The model under review builds one solid part; all positions refer to its coordinate system, in mm. A direction names the side the tool comes from. Give positions to 0.01 mm unless a question says otherwise; leave off trailing zeros. Loops run counter-clockwise (first coordinate to the right, second up) from the corner with the lowest first, then second, coordinate; pieces in that order, holes last. Notation, with made-up numbers: M 10,-28.5 L 16,-28.5 A16 cw 16,-1.5 Z; hole C 77,66.25 d11. An arc over 180 degrees is marked long. One line per item, written item: value. Start each with the question number.
Q1. We need section B-B on x = -7. Write out the cut boundary in (y, z).
Q2. We need section A-A on x = 0. Write out the cut boundary in (y, z).
Q3. For faces 4 (the face through (-10.011, 0.74, 10.124)), 5 (the face through (4.052, 4.986, -2.324)), 6 (the face through (-4.032, 3, 0)), list the 3-axis set-ups (+Z, -Z, +X, -X, +Y, -Y) from which the entire face can be reached by the end or side of a thin tool; tool diameter is ignored.
Q4. We need section D-D on x = 15. Write out the cut boundary in (y, z), plus the area to 3 significant figures.
Q5. To check wall thickness, follow line 1 along Y through (x, z) = (-4, 0.5); line 2 along X through (y, z) = (0.7, 8.5); line 3 along Y through (x, z) = (19, 9.5). State the ranges of each line that lie inside material, in increasing order. Write a range as from..to.
Q6. For pin 1 (1 mm diameter, centred on x = 19.5, z = -9, fed in from -Y); pin 2 (0.6 mm diameter, centred on y = 5.5, z = -2.5, fed in from -X); pin 3 (1 mm diameter, centred on y = 4.5, z = 8.5, fed in from +X); pin 4 (1 mm diameter, centred on x = -6.5, y = 4.5, fed in from -Z), all flat-tipped, find the tip position at first contact; note any pin that passes through.
Q7. Mouldability with a two-part tool opening along X and no side actions: class faces 1 (the face through (0, 1, -11.5)), 2 (the face through (3.815, 4.986, 3.181)), 3 (the face through (5.098, 5, 0)) as released by +X, released by -X, zero draft, split by the parting line, or undercut.
Q8. We need section C-C on y = 4.8. Write out the cut boundary in (x, z), plus the area to 3 significant figures.
```python
from build123d import *

# Parameters (mm, degrees)
SKETCH_1_W      = 51
SKETCH_1_H      = 23
SKETCH_1_R      = 0.5
SKETCH_1_R_2    = 1
EXTRUDE_1_DEPTH = 1.5
SKETCH_2_W      = 18.258727374
SKETCH_2_H      = 13.578190662
EXTRUDE_2_DEPTH = 2.5
SKETCH_3_W      = 29.608747094
SKETCH_3_H      = 20
SKETCH_3_R      = 0.75
EXTRUDE_3_DEPTH = 2


with BuildPart() as part:
    # Эскиз1 → Бобышка-Вытянуть1 (new body)
    with BuildSketch(Plane(origin=(0, 0, 0), x_dir=(1, 0, 0), z_dir=(0, 1, 0))):
        Rectangle(SKETCH_1_W, SKETCH_1_H)
        with Locations(Location((-18.598557526, 8.885912105, 0), (0, 0, 270))):
            Circle(SKETCH_1_R, mode=Mode.SUBTRACT)
        with Locations(Location((18.886719194, 8.885912105, 0), (0, 0, 270))):
            Circle(SKETCH_1_R_2, mode=Mode.SUBTRACT)
        with Locations(Location((22.095575567, -3.293156401, 0), (0, 0, 270))):
            Circle(SKETCH_1_R_2, mode=Mode.SUBTRACT)
        with Locations(Location((22.095575567, 1.301342497, 0), (0, 0, 270))):
            Circle(SKETCH_1_R_2, mode=Mode.SUBTRACT)
        with Locations(Location((7.364007673, -9.200369269, 0), (0, 0, 270))):
            Circle(SKETCH_1_R_2, mode=Mode.SUBTRACT)
        with Locations(Location((-9.628345393, -9.200369269, 0), (0, 0, 270))):
            Circle(SKETCH_1_R_2, mode=Mode.SUBTRACT)
    extrude(amount=EXTRUDE_1_DEPTH)

    # Эскиз2 → Бобышка-Вытянуть2 (add)
    with BuildSketch(Plane(origin=(0, 1.5, 0), x_dir=(1, 0, 0), z_dir=(0, 1, 0))):
        with Locations((-13.161113133, 0)):
            Rectangle(SKETCH_2_W, SKETCH_2_H)
    extrude(amount=EXTRUDE_2_DEPTH)

    # Эскиз3 → Бобышка-Вытянуть3 (add)
    with BuildSketch(Plane(origin=(0, 4, 0), x_dir=(1, 0, 0), z_dir=(0, 1, 0))):
        with Locations((-9.706759305, 0)):
            Rectangle(SKETCH_3_W, SKETCH_3_H)
        with Locations(Location((3.308209816, -7.836846056, 0), (0, 0, 270))):
            Circle(SKETCH_3_R, mode=Mode.SUBTRACT)
        with Locations(Location((3.308209816, -3.733593915, 0), (0, 0, 270))):
            Circle(SKETCH_3_R, mode=Mode.SUBTRACT)
        Polygon((-4.031749446, 0), (-4.031749446, -6.789095331), (-22.29047682, -6.789095331), (-22.29047682, 6.789095331), (-4.031749446, 6.789095331), align=None, mode=Mode.SUBTRACT)
        with Locations(Location((3.308209816, 2.226781891, 0), (0, 0, 270))):
            Circle(SKETCH_3_R, mode=Mode.SUBTRACT)
        with Locations(Location((3.308209816, 6.789095331, 0), (0, 0, 270))):
            Circle(SKETCH_3_R, mode=Mode.SUBTRACT)
        Polygon((-22.29047682, 6.789095331), (-13.161113133, 0), (-4.031749446, 6.789095331), align=None)
        Polygon((-22.29047682, 6.789095331), (-22.29047682, -6.789095331), (-13.161113133, 0), align=None)
        Polygon((-22.29047682, -6.789095331), (-4.031749446, -6.789095331), (-13.161113133, 0), align=None)
        Polygon((-13.161113133, 0), (-4.031749446, -6.789095331), (-4.031749446, 0), align=None)
        Polygon((-4.031749446, 6.789095331), (-13.161113133, 0), (-4.031749446, 0), align=None)
    extrude(amount=EXTRUDE_3_DEPTH)


solid = part.part
```
Solved:
1. outline: M 0,-11.5 L 1.5,-11.5 L 1.5,-6.79 L 4,-6.79 L 4,-10 L 6,-10 L 6,10 L 4,10 L 4,6.79 L 1.5,6.79 L 1.5,11.5 L 0,11.5 Z
2. outline: M 0,-11.5 L 1.5,-11.5 L 1.5,11.5 L 0,11.5 Z; M 4,-10 L 6,-10 L 6,10 L 4,10 Z
3. face 4: -Y
3. face 5: +Y
3. face 6: +Z, -Z, +X
4. outline: M 0,-11.5 L 1.5,-11.5 L 1.5,11.5 L 0,11.5 Z
4. area: 34.5 mm2
5. line 1: 0..1.5, 4..6
5. line 2: -25.5..-10.34, -8.91..6.65, 8.08..25.5
5. line 3: 0..1.5
6. pin 1: y = 0
6. pin 2: x = -24.51
6. pin 3: x = 5.1
6. pin 4: z = -10
7. face 1: zero draft
7. face 2: undercut
7. face 3: released by +X
8. outline: M -24.51,-10 L 5.1,-10 L 5.1,10 L -24.51,10 Z; hole C 3.31,-6.79 d1.5; hole C 3.31,-2.23 d1.5; hole C 3.31,3.73 d1.5; hole C 3.31,7.84 d1.5
8. area: 585 mm2
